Design review of the part built by this model. Coordinates are the model's own, in mm. Face numbers are marked on the shaded views. A direction names the side the tool comes from. Coordinates: 2 decimals unless noted, no trailing zeros. Write each loop counter-clockwise with the first axis right and the second up, starting at its lowest first coordinate (ties: lowest second). Pieces come first, ordered by that corner, then holes. Notation, with made-up numbers: (-12, -3) - (40, -3) arc R21 cw to (40, 6) - close; hole circle Ø1 at (74, 30.25). An arc over 180 degrees is marked (long way). Answer as a JSON object with one key per item and string values.
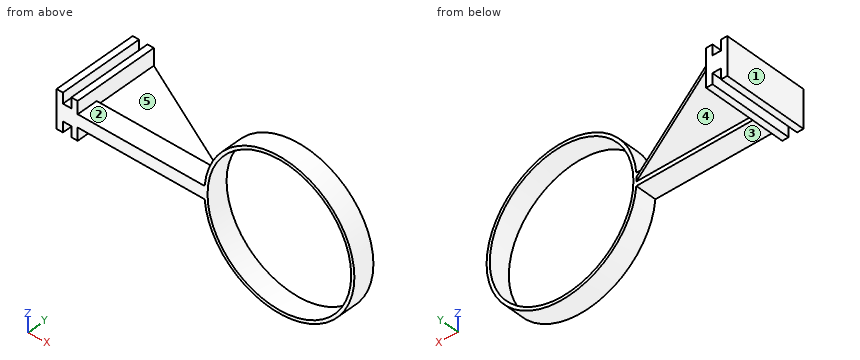
```python
from build123d import *

# Parameters (mm, degrees)
SKETCH8_R            = 17
BOSS_EXTRUDE10_DEPTH = 5
BOSS_EXTRUDE11_DEPTH = 20
BOSS_EXTRUDE13_START = -1
BOSS_EXTRUDE13_DEPTH = 1


with BuildPart() as part:
    # Sketch8 → Boss-Extrude10 (new body)
    with BuildSketch(Plane(origin=(0, 0, 0), x_dir=(1, 0, 0), z_dir=(0, 1, 0))):
        with BuildLine():
            Line((-17.686506156, 1.5), (-47.720151855, 1.5))
            Line((-47.720151855, 1.5), (-47.720151855, -1.5))
            Line((-47.720151855, -1.5), (-17.686506156, -1.5))
            ThreePointArc((-17.686506156, -1.5), (17.75, 0), (-17.686506156, 1.5))
        make_face()
        with Locations(Location((0, 0, 0), (0, 0, 270))):
            Circle(SKETCH8_R, mode=Mode.SUBTRACT)
    extrude(amount=BOSS_EXTRUDE10_DEPTH)

    # Sketch8_3 → Boss-Extrude11 (add)
    with BuildSketch(Plane(origin=(0, 0, 0), x_dir=(1, 0, 0), z_dir=(0, 1, 0))):
        Polygon((-47.720151855, -1.5), (-47.720151855, 1.5), (-47.720151855, 4.5), (-49.220151855, 4.5), (-49.220151855, 2), (-51.220151855, 2), (-51.220151855, 4.5), (-52.720151855, 4.5), (-52.720151855, -4.5), (-51.220151855, -4.5), (-51.220151855, -2), (-49.220151855, -2), (-49.220151855, -4.5), (-47.720151855, -4.5), align=None)
    extrude(amount=BOSS_EXTRUDE11_DEPTH)

    # Sketch9 → Boss-Extrude13 (add)
    with BuildSketch(Plane.XY.offset(1.5).offset(BOSS_EXTRUDE13_START)):
        Polygon((-17.686506156, 5), (-47.720151855, 5), (-47.720151855, 20), align=None)
    extrude(amount=-BOSS_EXTRUDE13_DEPTH)


solid = part.part
```
(1) Tool access review of the marked faces 1, 2, 3, 4 and 5: name each direction out of +Z, -Z, +X, -X, +Y, -Y from which nothing blocks a thin tool from reaching the whole face with its end or side.
Solved:
{"face 1": "+Z, -Z, -X, +Y, -Y", "face 2": "+Z, +Y, -Y", "face 3": "-Z, +Y, -Y", "face 4": "-Z, +X, +Y", "face 5": "+Z, +X, +Y"}
(2) Take a section at A-A, the plane x = 0. Write out the cut boundary in (y, z).
Solved:
{"outline": "(0, -17.75) - (5, -17.75) - (5, -17) - (0, -17) - close; (0, 17) - (5, 17) - (5, 17.75) - (0, 17.75) - close"}
(3) To check wall thickness, follow line 1 (X direction, y = 3.4, z = 0); line 2 (X direction, y = 4, z = -3); line 3 (X direction, y = 4.5, z = 3.5). State the ranges of each line that lie inside material, in increasing order. Write a range as from..to.
Solved:
{"line 1": "x = -52.72..-17, 17..17.75", "line 2": "x = -52.72..-51.22, -49.22..-47.72, -17.49..-16.73, 16.73..17.49", "line 3": "x = -52.72..-51.22, -49.22..-47.72, -17.4..-16.64, 16.64..17.4"}
(4) Take a section at B-B, the plane z = 13. Write out the cut boundary in (x, y), and give its area (3 significant figures).
Solved:
{"outline": "(-12.09, 0) - (-10.95, 0) - (-10.95, 5) - (-12.09, 5) - close; (10.95, 0) - (12.09, 0) - (12.09, 5) - (10.95, 5) - close", "area": "11.3 mm^2"}
(5) Take a section at C-C, the plane y = 18.25. Write out the cut boundary in (x, z).
Solved:
{"outline": "(-52.72, -4.5) - (-51.22, -4.5) - (-51.22, -2) - (-49.22, -2) - (-49.22, -4.5) - (-47.72, -4.5) - (-47.72, -0.5) - (-44.22, -0.5) - (-44.22, 0.5) - (-47.72, 0.5) - (-47.72, 4.5) - (-49.22, 4.5) - (-49.22, 2) - (-51.22, 2) - (-51.22, 4.5) - (-52.72, 4.5) - close"}
(6) Take a section at D-D, the plane x = -45. Write out the cut boundary in (y, z), and give its area (3 significant figures).
Solved:
{"outline": "(0, -1.5) - (5, -1.5) - (5, -0.5) - (18.64, -0.5) - (18.64, 0.5) - (5, 0.5) - (5, 1.5) - (0, 1.5) - close", "area": "28.6 mm^2"}
(7) For pin 1 (1.2 mm diameter, centred on x = -48.5, y = 13.5, fed in from -Z); pin 2 (1.2 mm diameter, centred on y = 6, z = 3, fed in from +X); pin 3 (5.5 mm diameter, centred on x = -38, y = 3, fed in from -Z); pin 4 (8 mm diameter, centred on y = 16.5, z = 10, fed in from -X), all flat-tipped, find the tip position at first contact; note any pin that passes through.
Solved:
{"pin 1": "stops at z = -4.5", "pin 2": "stops at x = -47.72", "pin 3": "stops at z = -1.5", "pin 4": "passes through"}
